from build123d import *

# Parameters (mm, degrees)
F0_W          = 12
F0_H          = 15
F2_R          = 2.54
F3_W          = 8.255
F3_H          = 1.6129
F4_DEPTH      = 12.7
F6_DEPTH      = 12.7
F8_DEPTH      = 5.08
F8_DEPTH_BACK = 25.4
F10_DEPTH     = 1.6129
F12_DEPTH     = 6.35
F13_R         = 1.190625
F14_DEPTH     = 1.5875
F15_R         = 1.190625
F16_DEPTH     = 1.5875
F17_R         = 1.190625
F18_DEPTH     = 1.5875
F19_R         = 3.175
F20_DEPTH     = 19.05


with BuildPart() as f1:
    # F0 (on Front) → F1 (revolve)
    with BuildSketch(Plane.XZ):
        with Locations((-6, 7.5)):
            Rectangle(F0_W, F0_H)
    revolve(axis=Axis((0, 0, 7.5), (0, 0, -1)))

    # F2
    f2_edges = [f1.edges().sort_by_distance(p)[0] for p in [
        (12, 0, 0),
    ]]
    fillet(f2_edges, radius=F2_R)

    # F3 (on Front) → F4 (cut, symmetric)
    with BuildSketch(Plane.XZ):
        with Locations((-4.1275, 12.60605)):
            Rectangle(F3_W, F3_H)
        with Locations((4.1275, 12.60605)):
            Rectangle(F3_W, F3_H)
    extrude(amount=F4_DEPTH, both=True, mode=Mode.SUBTRACT)

    # F5 (on Right) → F6 (cut, symmetric)
    with BuildSketch(Plane.YZ):
        Polygon((6.1694761611, 13.4125), (-6.1694761611, 13.4125), (-6.1694761611, 11.7996), (0, 11.7996), (6.1694761611, 11.7996), align=None)
    extrude(amount=F6_DEPTH, both=True, mode=Mode.SUBTRACT)

    # F7 (on Front) → F8 (cut, two sides)
    with BuildSketch(Plane.XZ) as f8_sk:
        Polygon((0, 11.7996), (-6.0325, 11.7996), (-6.0325, 9.41835), (6.0325, 9.41835), (6.0325, 11.7996), align=None)
    extrude(amount=-F8_DEPTH, mode=Mode.SUBTRACT)
    extrude(f8_sk.sketch, amount=F8_DEPTH_BACK, mode=Mode.SUBTRACT)

    # F9 (on face) → F10 (join)
    with BuildSketch(Plane.XY.offset(11.7996)):
        with BuildLine():
            Line((0, 10.984), (-8.255, 10.984))
            Line((-8.255, 10.984), (-8.255, -11.9694016141))
            ThreePointArc((-8.255, -11.9694016141), (0, -14.54), (8.255, -11.9694016141))
            Line((8.255, -11.9694016141), (8.255, 10.984))
            Line((8.255, 10.984), (0, 10.984))
        make_face()
    extrude(amount=F10_DEPTH)

    # F11 (on face) → F12 (join)
    with BuildSketch(Plane.XY.offset(13.4125)):
        with BuildLine():
            ThreePointArc((6.7911445407, -12.8565919212), (5.8958664247, -13.2909878904), (4.972972884, -13.6631307062))
            ThreePointArc((4.972972884, -13.6631307062), (4.0267866244, -13.9712773032), (3.0617394519, -14.213984365))
            Line((3.0617394519, -14.213984365), (3.6046964295, -15.7057464005))
            Line((3.6046964295, -15.7057464005), (7.3341015182, -14.3483539567))
            Line((7.3341015182, -14.3483539567), (6.7911445407, -12.8565919212))
        make_face()
        with BuildLine():
            ThreePointArc((1.984375, -14.4039527859), (0.9945165892, -14.5059483231), (0, -14.54))
            ThreePointArc((0, -14.54), (-0.9945165892, -14.5059483231), (-1.984375, -14.4039527859))
            Line((-1.984375, -14.4039527859), (-1.984375, -15.9914527859))
            Line((-1.984375, -15.9914527859), (1.984375, -15.9914527859))
            Line((1.984375, -15.9914527859), (1.984375, -14.4039527859))
        make_face()
        with BuildLine():
            ThreePointArc((-3.0617394519, -14.213984365), (-4.972972884, -13.6631307062), (-6.7911445407, -12.8565919212))
            Line((-6.7911445407, -12.8565919212), (-7.3341015182, -14.3483539567))
            Line((-7.3341015182, -14.3483539567), (-3.6046964295, -15.7057464005))
            Line((-3.6046964295, -15.7057464005), (-3.0617394519, -14.213984365))
        make_face()
    extrude(amount=-F12_DEPTH)

    # F13 (on face) → F14 (cut, through all)
    with BuildSketch(Plane(origin=(5.4693989738, -15.0270501786, 0), x_dir=(0.9396926208, 0.3420201433, 0), z_dir=(0.3420201433, -0.9396926208, 0))):
        with BuildLine():
            ThreePointArc((-1.984375, 9.046875), (-1.6602472402, 10.13376195), (-0.79375, 10.8655847289))
            Line((-0.79375, 10.8655847289), (-0.79375, 13.4125))
            Line((-0.79375, 13.4125), (-1.984375, 13.4125))
            Line((-1.984375, 13.4125), (-1.984375, 9.046875))
        make_face()
        with BuildLine():
            ThreePointArc((0.79375, 10.8655847289), (1.6602472402, 10.13376195), (1.984375, 9.046875))
            Line((1.984375, 9.046875), (1.984375, 13.4125))
            Line((1.984375, 13.4125), (0.79375, 13.4125))
            Line((0.79375, 13.4125), (0.79375, 10.8655847289))
        make_face()
        with BuildLine():
            Line((1.984375, 7.0625), (1.984375, 9.046875))
            ThreePointArc((1.984375, 9.046875), (1.4031650189, 7.6437099811), (0, 7.0625))
            Line((0, 7.0625), (1.984375, 7.0625))
        make_face()
        with BuildLine():
            Line((-1.984375, 7.0625), (0, 7.0625))
            ThreePointArc((0, 7.0625), (-1.4031650189, 7.6437099811), (-1.984375, 9.046875))
            Line((-1.984375, 9.046875), (-1.984375, 7.0625))
        make_face()
        with Locations((0, 9.046875)):
            Circle(F13_R)
    extrude(amount=-F14_DEPTH, mode=Mode.SUBTRACT)

    # F15 (on face) → F16 (cut, through all)
    with BuildSketch(Plane.XZ.offset(15.9914527859)):
        with BuildLine():
            ThreePointArc((-1.984375, 9.046875), (-1.6602472402, 10.13376195), (-0.79375, 10.8655847289))
            Line((-0.79375, 10.8655847289), (-0.79375, 13.4125))
            Line((-0.79375, 13.4125), (-1.984375, 13.4125))
            Line((-1.984375, 13.4125), (-1.984375, 9.046875))
        make_face()
        with BuildLine():
            ThreePointArc((0.79375, 10.8655847289), (1.6602472402, 10.13376195), (1.984375, 9.046875))
            Line((1.984375, 9.046875), (1.984375, 13.4125))
            Line((1.984375, 13.4125), (0.79375, 13.4125))
            Line((0.79375, 13.4125), (0.79375, 10.8655847289))
        make_face()
        with Locations((0, 9.046875)):
            Circle(F15_R)
        with BuildLine():
            Line((1.984375, 7.0625), (1.984375, 9.046875))
            ThreePointArc((1.984375, 9.046875), (1.4031650189, 7.6437099811), (0, 7.0625))
            Line((0, 7.0625), (1.984375, 7.0625))
        make_face()
        with BuildLine():
            Line((-1.984375, 7.0625), (0, 7.0625))
            ThreePointArc((0, 7.0625), (-1.4031650189, 7.6437099811), (-1.984375, 9.046875))
            Line((-1.984375, 9.046875), (-1.984375, 7.0625))
        make_face()
    extrude(amount=-F16_DEPTH, mode=Mode.SUBTRACT)

    # F17 (on face) → F18 (cut, through all)
    with BuildSketch(Plane(origin=(-5.4693989738, -15.0270501786, 0), x_dir=(0.9396926208, -0.3420201433, 0), z_dir=(-0.3420201433, -0.9396926208, 0))):
        with BuildLine():
            ThreePointArc((-1.984375, 9.046875), (-1.6602472402, 10.13376195), (-0.79375, 10.8655847289))
            Line((-0.79375, 10.8655847289), (-0.79375, 13.4125))
            Line((-0.79375, 13.4125), (-1.984375, 13.4125))
            Line((-1.984375, 13.4125), (-1.984375, 9.046875))
        make_face()
        with BuildLine():
            ThreePointArc((0.79375, 10.8655847289), (1.6602472402, 10.13376195), (1.984375, 9.046875))
            Line((1.984375, 9.046875), (1.984375, 13.4125))
            Line((1.984375, 13.4125), (0.79375, 13.4125))
            Line((0.79375, 13.4125), (0.79375, 10.8655847289))
        make_face()
        with Locations((0, 9.046875)):
            Circle(F17_R)
        with BuildLine():
            Line((1.984375, 7.0625), (1.984375, 9.046875))
            ThreePointArc((1.984375, 9.046875), (1.4031650189, 7.6437099811), (0, 7.0625))
            Line((0, 7.0625), (1.984375, 7.0625))
        make_face()
        with BuildLine():
            Line((-1.984375, 7.0625), (0, 7.0625))
            ThreePointArc((0, 7.0625), (-1.4031650189, 7.6437099811), (-1.984375, 9.046875))
            Line((-1.984375, 9.046875), (-1.984375, 7.0625))
        make_face()
    extrude(amount=-F18_DEPTH, mode=Mode.SUBTRACT)

    # F19 (on face) → F20 (join)
    with BuildSketch(Plane.XY.offset(15)):
        Circle(F19_R)
    extrude(amount=F20_DEPTH)

    # F21 (on Front) → F22 (revolve)
    with BuildSketch(Plane.XZ):
        with BuildLine():
            Line((0, 38.8125), (0, 34.05))
            Line((0, 34.05), (3.048, 34.05))
            ThreePointArc((3.048, 34.05), (2.651125, 34.446875), (3.048, 34.84375))
            Line((3.048, 34.84375), (3.175, 34.84375))
            Line((3.175, 34.84375), (2.54, 38.8125))
            Line((2.54, 38.8125), (0, 38.8125))
        make_face()
    revolve(axis=Axis((0, 0, 36.43125), (0, 0, 1)))


solid = f1.part
Design review of the part built by this model. Coordinates are the model's own, in mm. A direction names the side the tool comes from. Round coordinates to 2 decimals unless told otherwise and drop trailing zeros. Write each loop counter-clockwise with the first axis right and the second up, starting at its lowest first coordinate (ties: lowest second). Pieces come first, ordered by that corner, then holes. Notation, with made-up numbers: (87.5, 32.25) -> (146.5, 32.25) arc R26 cw to (146.5, 61.25) -> close; hole circle Ø8 at (51.25, -20). An arc over 180 degrees is marked (long way). One line per question, with ' | ' between items.
(1) Take a section at C-C, the plane z = 24. State the section outline as (x, y) points (3 decimals), and give its area (3 significant figures).
Result sheet:
outline: circle Ø6.35 at (0, 0) | area: 31.7 mm2
(2) Insertion check: P1, Ø1.3, axis at x = 9, z = 13, coming from the +Y side; P2, Ø1.8, axis at y = 10.5, z = 12.5, coming from the -X side (3 decimals); P3, Ø4, axis at x = -11, y = -3, coming from the +Z side; P4, Ø1, axis at x = 4.5, z = 19, coming from the -Y side. Each pin has a flat end and moves straight along its axis. Give the tip position at first contact, or say it passes through.
Result sheet:
P1: y = 8.62 | P2: x = -8.255 | P3: z = 15 | P4: through
(3) Draft analysis for pull direction Z (two halves, no side actions). For faces 1 (the flat face through (-3.629, -14.008, 12.617)), 2 (the cylindrical face through (-0.88, -15.25, 9.85)), 3 (the flat face through (-0.1, -12.3, 13.412)), 4 (the flat face through (7, 10, 11.8)), state which applies: released by +Z, released by -Z, zero draft, split by the parting line, or undercut.
Result sheet:
face 1: zero draft | face 2: undercut | face 3: released by +Z | face 4: released by -Z
(4) Take a section at B-B, the plane z = 36. State the section outline as (x, y) points, and give its area (3 significant figures).
Result sheet:
outline: circle Ø5.98 at (0, 0) | area: 28.1 mm2
(5) Wall thickness on line 1 (Z direction, x = 0, y = -15.55); line 2 (Z direction, x = -3.25, y = 0.75); line 3 (Z direction, x = 6.5, y = 4): over which ranges is each line inside the solid? List them lowest first. Write a range as [from, to].
Result sheet:
line 1: [7.06, 7.86], [10.24, 13.41] | line 2: [0, 9.42], [11.8, 15] | line 3: [0, 15]
(6) Machinability: for faces 5 (the flat face through (6.032, -3, 11)), 6 (the cylindrical face through (2.52, -14.32, 12.59)), 7 (the cylindrical face through (-0.69, -3.1, 24.39)), 8 (the flat face through (-7, 10, 13.412)), which of the approach directions +Z, -Z, +X, -X, +Y, -Y give a long, thin tool a straight path to every point of the face, cutting with its end or side? Answer none if there is none.
Result sheet:
face 5: none | face 6: +Z, -Z, -Y | face 7: +Z | face 8: +Z, -X, +Y
